CAD build for the part. Positions are in the model's coordinates, mm. A direction names the side the tool comes from. Round coordinates to 2 decimals unless told otherwise and drop trailing zeros. Loops run counter-clockwise (first coordinate to the right, second up) from the corner with the lowest first, then second, coordinate; pieces in that order, holes last.
from build123d import *

# Parameters (mm, degrees)
BOSS_EXTRUDE1_DEPTH = 25
CUT_EXTRUDE1_DEPTH  = 5
SKETCH3_R           = 1.75
CUT_EXTRUDE2_DEPTH  = 5


with BuildPart() as part:
    # Sketch1 → Boss-Extrude1 (new body)
    with BuildSketch(Plane(origin=(0, 0, 0), x_dir=(1, 0, 0), z_dir=(0, 1, 0))):
        Polygon((-5, 15), (-5, -5), (15, -5), (15, 0), (0, 0), (0, 15), align=None)
    extrude(amount=BOSS_EXTRUDE1_DEPTH)

    # Sketch2 → Cut-Extrude1 (cut)
    with BuildSketch(Plane(origin=(0, 0, 0), x_dir=(-1, 0, 0), z_dir=(0, 0, -1))):
        with BuildLine():
            Line((-7.75, 20.5), (-7.75, 4.5))
            ThreePointArc((-7.75, 4.5), (-9.5, 2.75), (-11.25, 4.5))
            Line((-11.25, 4.5), (-11.25, 20.5))
            ThreePointArc((-11.25, 20.5), (-9.5, 22.25), (-7.75, 20.5))
        make_face()
    extrude(amount=-CUT_EXTRUDE1_DEPTH, mode=Mode.SUBTRACT)

    # Sketch3 → Cut-Extrude2 (cut)
    with BuildSketch(Plane.ZY.offset(5)):
        with Locations((-5, 5.134)):
            Circle(SKETCH3_R)
        with Locations((-5, 19.866)):
            Circle(SKETCH3_R)
    extrude(amount=-CUT_EXTRUDE2_DEPTH, mode=Mode.SUBTRACT)


solid = part.part
Item 1: 3-axis set-ups, long thin cutter, end or side, ignore diameter. For faces 1 (the flat face through (-2, 0, -1)), 2 (the flat face through (7.75, 13, 2)), 3 (the flat face through (0, 12, -7)): which of +Z, -Z, +X, -X, +Y, -Y reach the whole face in a straight line?
Verdict:
face 1: +Z, -Z, +X, -X, -Y
face 2: +Z, -Z
face 3: -Z, +X, +Y, -Y
Item 2: Mould opens along Y. For faces 4 (the cylindrical face through (-2.54, 5.21, -6.75)), 5 (the flat face through (-2, 25, -1)), 6 (the flat face through (15, 12, 3)) say: released by +Y, released by -Y, zero draft, split by the parting line, or undercut.
Verdict:
face 4: undercut
face 5: released by +Y
face 6: zero draft
Item 3: Cut at C-C (x = 9.5). List the corners of the cut face in (y, z).
Verdict:
outline: (0, 0) - (2.75, 0) - (2.75, 5) - (0, 5) - close; (22.25, 0) - (25, 0) - (25, 5) - (22.25, 5) - close
Item 4: Cut at D-D (y = 19.5). List the corners of the cut face in (x, z).
Verdict:
outline: (-5, -15) - (0, -15) - (0, -6.71) - (-5, -6.71) - close; (-5, -3.29) - (0, -3.29) - (0, 0) - (7.75, 0) - (7.75, 5) - (-5, 5) - close; (11.25, 0) - (15, 0) - (15, 5) - (11.25, 5) - close
Item 5: Wall check: L1, parallel to Y at x = -3.3, z = -5; L2, parallel to X at y = 22.5, z = -10.25; L3, parallel to Z at x = 5.5, y = 3.75. Give the ranges that are in metal, low to high.
Verdict:
L1: y = 0 to 3.38, 6.88 to 18.12, 21.62 to 25
L2: x = -5 to 0
L3: z = 0 to 5
Item 6: Flat gauge pins, fed straight in: P1, Ø12, axis at x = 11, y = 17, coming from the -Z side; P2, Ø7.5, axis at y = 17, z = -11, coming from the +X side. Where does each tip first touch, or does it go through?
Verdict:
P1: stops at z = 0
P2: stops at x = 0
Item 7: Cut at B-B (y = 16). List the corners of the cut face in (x, z).
Verdict:
outline: (-5, -15) - (0, -15) - (0, 0) - (7.75, 0) - (7.75, 5) - (-5, 5) - close; (11.25, 0) - (15, 0) - (15, 5) - (11.25, 5) - close
Item 8: Cut at A-A (z = -5). List the corners of the cut face in (x, y), plus the area to 3 significant figures.
Verdict:
outline: (-5, 0) - (0, 0) - (0, 3.38) - (-5, 3.38) - close; (-5, 6.88) - (0, 6.88) - (0, 18.12) - (-5, 18.12) - close; (-5, 21.62) - (0, 21.62) - (0, 25) - (-5, 25) - close
area: 90.0 mm2
